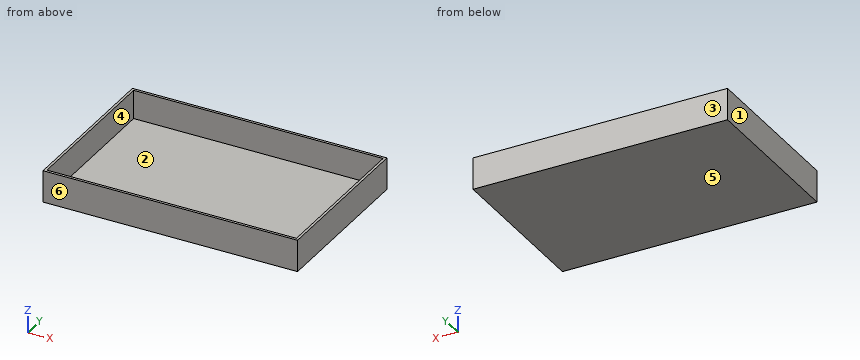
```python
from build123d import *

# Parameters (mm, degrees)
F0_W     = 800
F0_H     = 100
F1_DEPTH = 8
F2_W     = 500
F2_H     = 100
F3_DEPTH = 8
F4_W     = 792
F4_H     = 100
F4_W_2   = 8
F5_DEPTH = 8
F6_W     = 500
F6_H     = 100
F7_DEPTH = 8
F8_W     = 784
F8_H     = 500
F9_DEPTH = 10


with BuildPart() as f1:
    # F0 (on Front) → F1 (new body)
    with BuildSketch(Plane.XZ):
        Rectangle(F0_W, F0_H)
    extrude(amount=F1_DEPTH)

    # F2 (on face) → F3 (join)
    with BuildSketch(Plane.YZ.offset(400)):
        with Locations((250, 0)):
            Rectangle(F2_W, F2_H)
    extrude(amount=-F3_DEPTH)

    # F4 (on face) → F5 (join)
    with BuildSketch(Plane(origin=(0, 500, 0), x_dir=(-1, 0, 0), z_dir=(0, 1, 0))):
        with Locations((4, 0)):
            Rectangle(F4_W, F4_H)
        with Locations((-396, 0)):
            Rectangle(F4_W_2, F4_H)
    extrude(amount=F5_DEPTH)

    # F6 (on face) → F7 (join)
    with BuildSketch(Plane(origin=(-400, 0, 0), x_dir=(0, -1, 0), z_dir=(-1, 0, 0))):
        with Locations((-250, 0)):
            Rectangle(F6_W, F6_H)
    extrude(amount=-F7_DEPTH)

    # F8 (on face) → F9 (join)
    with BuildSketch(Plane(origin=(0, 0, -50), x_dir=(1, 0, 0), z_dir=(0, 0, -1))):
        with Locations((0, -250)):
            Rectangle(F8_W, F8_H)
    extrude(amount=-F9_DEPTH)


solid = f1.part
```
CAD build for the part. Positions are in the model's coordinates, mm. Face numbers are marked on the shaded views. A direction names the side the tool comes from. Round coordinates to 2 decimals unless told otherwise and drop trailing zeros. Loops run counter-clockwise (first coordinate to the right, second up) from the corner with the lowest first, then second, coordinate; pieces in that order, holes last. Notation, with made-up numbers: M 14.25,24.25 L 31.25,24.25 A31 ccw 31.25,49.25 Z; hole C -11,40 d10. An arc over 180 degrees is marked long. Return JSON: item names as keys, results as strings. Group by question number.
(1) Saw through at B-B, the plane y = 39. List the corners of the cut face in (x, z), and give its area (3 significant figures).
(2) Tool access for the marked faces 1 and 2: list every direction of +Z, -Z, +X, -X, +Y, -Y with a clear straight run to the whole face (end or side of a thin tool).
(3) Drop a flat-ended pin along its axis: P1, Ø3, axis at x = -88.5, y = 205.5, coming from the +Z side. Give the stop position or say it passes through.
(4) Saw through at C-C, the plane x = 174.5. List the corners of the cut face in (y, z), and give its area (3 significant figures).
(5) Mould opens along Y. For the marked faces 3, 4, 5 and 6 say: +Y half, -Y half, draft (parallel to the pull), parting line (faces both ways), or undercut.
(6) Saw through at A-A, the plane z = 6. List the corners of the cut face in (x, y), and give its area (3 significant figures).
(7) Wall check: probe 1 along Y at (x, z) = (142.5, 44); probe 2 along X at (y, z) = (308, 42.5); probe 3 along Z at (x, y) = (-184.5, 280). Give the ranges that are in metal, low to high. Write a range as [from, to].
Answer list:
{
 "1": {"outline": "M -400,-50 L 400,-50 L 400,50 L 392,50 L 392,-40 L -392,-40 L -392,50 L -400,50 Z", "area": "9,440 mm2"},
 "2": {"face 1": "+Z, -Z, -X, +Y, -Y", "face 2": "+Z"},
 "3": {"P1": "z = -40"},
 "4": {"outline": "M -8,-50 L 508,-50 L 508,50 L 500,50 L 500,-40 L 0,-40 L 0,50 L -8,50 Z", "area": "6,600 mm2"},
 "5": {"face 3": "+Y half", "face 4": "undercut", "face 5": "draft", "face 6": "-Y half"},
 "6": {"outline": "M -400,-8 L 400,-8 L 400,508 L -400,508 Z; hole M -392,0 L 392,0 L 392,500 L -392,500 Z", "area": "20,800 mm2"},
 "7": {"probe 1": "[-8, 0], [500, 508]", "probe 2": "[-400, -392], [392, 400]", "probe 3": "[-50, -40]"}
}
